For this review, take the finished solid that the model builds, in its own axes (mm). A direction names the side the tool comes from. Give positions to 0.01 mm unless a question says otherwise; leave off trailing zeros. Write each loop counter-clockwise with the first axis right and the second up, starting at its lowest first coordinate (ties: lowest second). Pieces come first, ordered by that corner, then holes. Notation, with made-up numbers: (-24.5, 8) -> (10.5, 8) arc R27 cw to (10.5, 34) -> close; hole circle Ø1 at (-28, 70). An arc over 180 degrees is marked (long way). Write item = value, one per line.
```python
from build123d import *

# Parameters (mm, degrees)
BOSS_EXTRU_1_DEPTH      = 7
ENL_V_MAT_EXTRU_1_DEPTH = 1.5
ESQUISSE3_R             = 1.75
ENL_V_MAT_EXTRU_2_DEPTH = 8.5
ESQUISSE4_W             = 12.5
ESQUISSE4_H             = 5
ENL_V_MAT_EXTRU_3_DEPTH = 9.2
BOSS_EXTRU_2_START      = 1.2
BOSS_EXTRU_2_DEPTH      = 1.8
BOSS_EXTRU_3_REACH      = 23.107
ESQUISSE8_W             = 0.2
ESQUISSE8_H             = 9.2
ESQUISSE6_R             = 4.379651067
ENL_V_MAT_EXTRU_4_DEPTH = 3
ENL_V_START             = 1
ESQUISSE7_R             = 4.166394869
ENL_V_MAT_EXTRU_5_DEPTH = 2
BOSS_EXTRU_4_START      = 1.5
ESQUISSE9_R             = 1.75
BOSS_EXTRU_4_DEPTH      = 1.5


with BuildPart() as part:
    # Esquisse1 → Boss.-Extru.1 (new, symmetric)
    with BuildSketch(Plane.XY):
        with BuildLine():
            Line((-15.5, 0), (-6.25, 0))
            Line((-6.25, 0), (-6.25, 5))
            ThreePointArc((-6.25, 5), (-5.590169944, 7.795084972), (-3.75, 10))
            Line((-3.75, 10), (3.75, 10))
            ThreePointArc((3.75, 10), (5.590169944, 7.795084972), (6.25, 5))
            Line((6.25, 5), (6.25, 0))
            Line((6.25, 0), (15.5, 0))
            Line((15.5, 0), (15.5, 4))
            Line((15.5, 4), (8.75, 4))
            Line((8.75, 4), (8.75, 12.5))
            Line((8.75, 12.5), (-8.75, 12.5))
            Line((-8.75, 12.5), (-8.75, 4))
            Line((-8.75, 4), (-15.5, 4))
            Line((-15.5, 4), (-15.5, 0))
        make_face()
    extrude(amount=BOSS_EXTRU_1_DEPTH, both=True)

    # Esquisse2 → Enlèv. mat.-Extru.1 (cut)
    with BuildSketch(Plane(origin=(0, 4, 0), x_dir=(1, 0, 0), z_dir=(0, 1, 0))):
        Polygon((-9.1, -1.674315781), (-9.1, 1.674315781), (-12, 3.348631561), (-14.9, 1.674315781), (-14.9, -1.674315781), (-12, -3.348631561), align=None)
        Polygon((9.1, -1.674315781), (12, -3.348631561), (14.9, -1.674315781), (14.9, 1.674315781), (12, 3.348631561), (9.1, 1.674315781), align=None)
    extrude(amount=-ENL_V_MAT_EXTRU_1_DEPTH, mode=Mode.SUBTRACT)

    # Esquisse3 → Enlèv. mat.-Extru.2 (cut)
    with BuildSketch(Plane(origin=(0, 2.5, 0), x_dir=(1, 0, 0), z_dir=(0, 1, 0))):
        with Locations(Location((-12, 0, 0), (0, 0, 270))):
            Circle(ESQUISSE3_R)
        with Locations(Location((12, 0, 0), (0, 0, 270))):
            Circle(ESQUISSE3_R)
    extrude(amount=-ENL_V_MAT_EXTRU_2_DEPTH, mode=Mode.SUBTRACT)

    # Esquisse4 → Enlèv. mat.-Extru.3 (cut)
    with BuildSketch(Plane(origin=(0, 0, -7), x_dir=(-1, 0, 0), z_dir=(0, 0, -1))):
        with Locations((0, 7.5)):
            Rectangle(ESQUISSE4_W, ESQUISSE4_H)
    extrude(amount=-ENL_V_MAT_EXTRU_3_DEPTH, mode=Mode.SUBTRACT)

    # Esquisse5 → Boss.-Extru.2 (add)
    with BuildSketch(Plane(origin=(0, 0, 2.2), x_dir=(-1, 0, 0), z_dir=(0, 0, -1)).offset(BOSS_EXTRU_2_START)):
        Polygon((-3.75, 10), (-6.25, 5), (-6.25, 10), align=None)
    extrude(amount=BOSS_EXTRU_2_DEPTH)

    # Boss.-Extru.3: up to this face of the body (flat: up to its plane)
    boss_extru_3_end = Plane(part.part.faces().sort_by_distance((-0.153583618, 10, -0.75665529))[0])
    # Esquisse8 → Boss.-Extru.3 (add, up to the picked face)
    with BuildSketch(Plane.XZ, mode=Mode.PRIVATE) as boss_extru_3_sk1:
        with Locations((6.15, -2.4)):
            Rectangle(ESQUISSE8_W, ESQUISSE8_H)
    boss_extru_3_tool1 = split(extrude(boss_extru_3_sk1.sketch, amount=-BOSS_EXTRU_3_REACH, mode=Mode.PRIVATE), bisect_by=boss_extru_3_end, keep=Keep.BOTH, mode=Mode.PRIVATE)
    # Esquisse8 → Boss.-Extru.3 (add, up to the picked face)
    with BuildSketch(Plane.XZ, mode=Mode.PRIVATE) as boss_extru_3_sk2:
        with Locations((-6.15, -2.4)):
            Rectangle(ESQUISSE8_W, ESQUISSE8_H)
    boss_extru_3_tool2 = split(extrude(boss_extru_3_sk2.sketch, amount=-BOSS_EXTRU_3_REACH, mode=Mode.PRIVATE), bisect_by=boss_extru_3_end, keep=Keep.BOTH, mode=Mode.PRIVATE)
    add(boss_extru_3_tool1.solids().sort_by(Axis((6.15, 0, -2.4), (0, 1, 0)))[0])
    add(boss_extru_3_tool2.solids().sort_by(Axis((-6.15, 0, -2.4), (0, 1, 0)))[0])

    # Esquisse6 → Enlèv. mat.-Extru.4 (cut)
    with BuildSketch(Plane.XY.offset(1)):
        with Locations((-2.786650878, 3.015494516)):
            Circle(ESQUISSE6_R)
    extrude(amount=-ENL_V_MAT_EXTRU_4_DEPTH, mode=Mode.SUBTRACT)

    # Esquisse7 → Enlèv. mat.-Extru.5 (cut)
    with BuildSketch(Plane(origin=(0, 0, -0.8), x_dir=(-1, 0, 0), z_dir=(0, 0, -1)).offset(ENL_V_START)):
        with Locations((-3.11839503, 6.498808114)):
            Circle(ESQUISSE7_R)
    extrude(amount=ENL_V_MAT_EXTRU_5_DEPTH, mode=Mode.SUBTRACT)

    # Esquisse9 → Boss.-Extru.4 (add)
    # profile 1 of 2: a face of its own
    with BuildSketch(Plane(origin=(0, 2.5, 0), x_dir=(1, 0, 0), z_dir=(0, 1, 0)).offset(BOSS_EXTRU_4_START)):
        Polygon((9.1, 1.674315781), (9.1, -1.674315781), (12, -3.348631561), (14.9, -1.674315781), (14.9, 1.674315781), (12, 3.348631561), align=None)
        with Locations(Location((12, 0, 0), (0, 0, 270))):
            Circle(ESQUISSE9_R, mode=Mode.SUBTRACT)
    # profile 2 of 2: a face of its own
    with BuildSketch(Plane(origin=(0, 2.5, 0), x_dir=(1, 0, 0), z_dir=(0, 1, 0)).offset(BOSS_EXTRU_4_START)):
        Polygon((-12, -3.348631561), (-9.1, -1.674315781), (-9.1, 1.674315781), (-12, 3.348631561), (-14.9, 1.674315781), (-14.9, -1.674315781), align=None)
        with Locations(Location((-12, 0, 0), (0, 0, 270))):
            Circle(ESQUISSE9_R, mode=Mode.SUBTRACT)
    extrude(amount=-BOSS_EXTRU_4_DEPTH)


solid = part.part
```
(1) The part is to be moulded in two halves that separate along Z. For faces 1 (the face through (13.735, 2.028, -0.228)), 2 (the face through (5, 9, 2.2)), 3 (the face through (-0.2, 10.3, -7)), 4 (the face through (-15.5, 2, 0)), say which applies: released by +Z, released by -Z, zero draft, split by the parting line, or undercut.
Answers below:
face_1 = undercut
face_2 = undercut
face_3 = released by -Z
face_4 = zero draft
(2) Tool access review of faces 5 (the face through (5.572, 7.831, 4.634)), 6 (the face through (7, 7, -1.8)), 7 (the face through (3.085, 10.665, -2.786)), 8 (the face through (-13, 4, 2)): name each direction out of +Z, -Z, +X, -X, +Y, -Y from which nothing blocks a thin tool from reaching the whole face with its end or side.
Answers below:
face_5 = +Z, -Y
face_6 = none
face_7 = -Y
face_8 = +Z, -Z, -X, +Y
(3) Take a section at C-C (y = 2.25). Write out the cut boundary in (x, z), plus the area to 3 significant figures.
Answers below:
outline = (-15.5, -7) -> (-6.05, -7) -> (-6.05, -2) -> (-7.1, -2) -> (-7.1, 1) -> (-6.05, 1) -> (-6.05, 2.2) -> (-6.25, 2.2) -> (-6.25, 7) -> (-15.5, 7) -> close; (6.05, -7) -> (15.5, -7) -> (15.5, 7) -> (6.25, 7) -> (6.25, 2.2) -> (6.05, 2.2) -> close; hole circle Ø3.5 at (-12, 0); hole circle Ø3.5 at (12, 0)
area = 240 mm^2
(4) Take a section at D-D (z = -5.75). Write out the cut boundary in (x, y).
Answers below:
outline = (-15.5, 0) -> (-6.05, 0) -> (-6.05, 10) -> (6.05, 10) -> (6.05, 0) -> (15.5, 0) -> (15.5, 4) -> (8.75, 4) -> (8.75, 12.5) -> (-8.75, 12.5) -> (-8.75, 4) -> (-15.5, 4) -> close
(5) To check wall thickness, follow probe 1 along X at (y, z) = (3.05, 0); probe 2 along X at (y, z) = (2.25, -4.5); probe 3 along X at (y, z) = (1.45, 0). State the ranges of each line that lie inside material, in increasing order.
Answers below:
probe_1 = -15.5 to -13.75, -10.25 to -7.17, 6.05 to 10.25, 13.75 to 15.5
probe_2 = -15.5 to -6.05, 6.05 to 15.5
probe_3 = -15.5 to -13.75, -10.25 to -6.88, 6.05 to 10.25, 13.75 to 15.5
(6) For pin 1 (3 mm diameter, centred on y = 9, z = -4, fed in from +X); pin 2 (2 mm diameter, centred on x = 12, z = 3.5, fed in from +Y); pin 3 (3 mm diameter, centred on x = -11.5, z = -1.5, fed in from -Y); pin 4 (3.5 mm diameter, centred on x = 0.5, z = 1.5, fed in from -Y), all flat-tipped, find the tip position at first contact; note any pin that passes through.
Answers below:
pin_1 = 8.75
pin_2 = 4
pin_3 = 0
pin_4 = 10
(7) Take a section at A-A (x = 12). Write out the cut boundary in (y, z).
Answers below:
outline = (0, -7) -> (4, -7) -> (4, -1.75) -> (0, -1.75) -> close; (0, 1.75) -> (4, 1.75) -> (4, 7) -> (0, 7) -> close
(8) Take a section at B-B (z = 0). Write out the cut boundary in (x, y), plus the area to 3 significant figures.
Answers below:
outline = (-15.5, 0) -> (-13.75, 0) -> (-13.75, 4) -> (-15.5, 4) -> close; (-10.25, 0) -> (-6.05, 0) -> (-6.05, 0.09) arc R4.38 cw to (-6.05, 5.94) -> (-6.05, 10) -> (3.75, 10) -> (6.05, 5.4) -> (6.05, 0) -> (10.25, 0) -> (10.25, 4) -> (8.75, 4) -> (8.75, 12.5) -> (-8.75, 12.5) -> (-8.75, 4) -> (-10.25, 4) -> close; (13.75, 0) -> (15.5, 0) -> (15.5, 4) -> (13.75, 4) -> close
area = 125 mm^2
